Model file for the job. Use its own axes, mm. Face numbers are marked on the shaded views. A direction names the side the tool comes from. Round coordinates to 2 decimals unless told otherwise and drop trailing zeros. Loops run counter-clockwise (first coordinate to the right, second up) from the corner with the lowest first, then second, coordinate; pieces in that order, holes last. Notation, with made-up numbers: (-38, 46) - (-6, 46) arc R11 ccw to (-6, 64) - close; hole circle Ø9 at (68, 8). An arc over 180 degrees is marked (long way). Answer as a JSON object with one key per item and string values.
from build123d import *

# Parameters (mm, degrees)
SKETCH1_W           = 120
SKETCH1_H           = 180
BOSS_EXTRUDE1_DEPTH = 45
SKETCH3_W           = 114
SKETCH3_H           = 174
CUT_EXTRUDE1_DEPTH  = 40
SKETCH4_R           = 2.5
CUT_EXTRUDE2_DEPTH  = 5


with BuildPart() as part:
    # Sketch1 → Boss-Extrude1 (new body)
    with BuildSketch(Plane(origin=(0, 0, 0), x_dir=(1, 0, 0), z_dir=(0, 1, 0))):
        with Locations((60, 90)):
            Rectangle(SKETCH1_W, SKETCH1_H)
    extrude(amount=BOSS_EXTRUDE1_DEPTH)

    # Sketch3 → Cut-Extrude1 (cut)
    with BuildSketch(Plane(origin=(0, 45, 0), x_dir=(1, 0, 0), z_dir=(0, 1, 0))):
        with Locations((60, 90)):
            Rectangle(SKETCH3_W, SKETCH3_H)
    extrude(amount=-CUT_EXTRUDE1_DEPTH, mode=Mode.SUBTRACT)

    # Sketch4 → Cut-Extrude2 (cut)
    with BuildSketch(Plane(origin=(0, 5, 0), x_dir=(1, 0, 0), z_dir=(0, 1, 0))):
        with Locations(Location((10.3, 85.818636822, 0), (0, 0, 270))):
            Circle(SKETCH4_R)
        with Locations(Location((60, 7, 0), (0, 0, 270))):
            Circle(SKETCH4_R)
    extrude(amount=-CUT_EXTRUDE2_DEPTH, mode=Mode.SUBTRACT)


solid = part.part
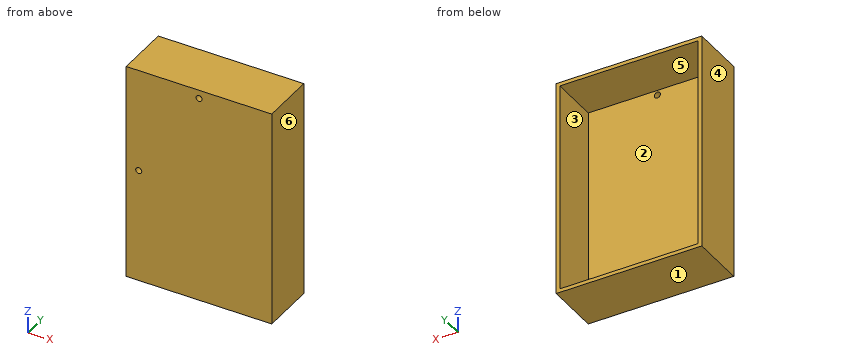
1) Slice it at D-D on z = -137.5. List the corners of the cut face in (x, y), then the cut area to 3 significant figures.
Values follow:
{"outline": "(0, 0) - (120, 0) - (120, 45) - (117, 45) - (117, 5) - (3, 5) - (3, 45) - (0, 45) - close", "area": "840 mm²"}
2) Slice it at A-A on z = -7. List the corners of the cut face in (x, y).
Values follow:
{"outline": "(0, 0) - (57.5, 0) - (57.5, 5) - (3, 5) - (3, 45) - (0, 45) - close; (62.5, 0) - (120, 0) - (120, 45) - (117, 45) - (117, 5) - (62.5, 5) - close"}
3) Slice it at B-B on x = 10.3. List the corners of the cut face in (y, z), then the cut area to 4 significant figures.
Values follow:
{"outline": "(0, -180) - (45, -180) - (45, -177) - (5, -177) - (5, -88.32) - (0, -88.32) - close; (0, -83.32) - (5, -83.32) - (5, -3) - (45, -3) - (45, 0) - (0, 0) - close", "area": "1,115 mm²"}
4) Slice it at C-C on y = 17.5. List the corners of the cut face in (x, z), then the cut area to 3 significant figures.
Values follow:
{"outline": "(0, -180) - (120, -180) - (120, 0) - (0, 0) - close; hole (3, -177) - (117, -177) - (117, -3) - (3, -3) - close", "area": "1,760 mm²"}
5) Probe probe 1 along Z at (x, y) = (33.5, 14); probe 2 along X at (y, z) = (22.5, -93); probe 3 along X at (y, z) = (1.75, -7). List the from-to ranges inside material, lowest first.
Values follow:
{"probe 1": "-180 to -177, -3 to 0", "probe 2": "0 to 3, 117 to 120", "probe 3": "0 to 57.5, 62.5 to 120"}
6) Drop a flat-ended pin along its axis: P1, Ø5, axis at x = 46.5, z = -24.5, coming from the +Y side. Give the stop position or say it passes through.
Values follow:
{"P1": "y = 5"}
7) Tool access for the marked faces 5 and 6: list every direction of +Z, -Z, +X, -X, +Y, -Y with a clear straight run to the whole face (end or side of a thin tool).
Values follow:
{"face 5": "+Y", "face 6": "+Z, -Z, +X, +Y, -Y"}
8) Two-plate mould, pull along Z, no slides. Class the marked faces 1, 2, 3 and 4: pulls with the +Z half, pulls with the -Z half, needs draft (parallel to the pull), parting line crosses it, or undercut.
Values follow:
{"face 1": "pulls with the -Z half", "face 2": "undercut", "face 3": "undercut", "face 4": "needs draft"}
